```python
from build123d import *

# Parameters (mm, degrees)
BOSS_EXTRUDE1_DEPTH = 45.72
CUT_EXTRUDE1_REACH  = 94.812
SKETCH2_R           = 12.7
SKETCH4_R           = 19.05
CUT_EXTRUDE2_DEPTH  = 2.54
SKETCH5_R           = 1.651
CUT_EXTRUDE3_DEPTH  = 94.150493289
FILLET1_R           = 0.508


with BuildPart() as part:
    # Sketch1 → Boss-Extrude1 (new body)
    with BuildSketch(Plane.XY):
        Polygon((13.1, 7.855), (5.48, 7.855), (5.48, 3.81), (80.52, 3.81), (80.52, 7.855), (72.9, 7.855), (72.9, 10.16), (13.1, 10.16), align=None)
    extrude(amount=-BOSS_EXTRUDE1_DEPTH)

    # Sketch2 → Cut-Extrude1 (cut, up to next)
    with BuildSketch(Plane.XZ.offset(-3.81), mode=Mode.PRIVATE) as cut_extrude1_sk1:
        with Locations(Location((43, -22.86, 0), (0, 0, 270))):
            Circle(SKETCH2_R)
    cut_extrude1_tool1 = extrude(cut_extrude1_sk1.sketch, amount=-CUT_EXTRUDE1_REACH, mode=Mode.PRIVATE) & part.part
    add(cut_extrude1_tool1.solids().sort_by_distance((43, 3.81, -22.86))[0], mode=Mode.SUBTRACT)

    # Sketch4 → Cut-Extrude2 (cut)
    with BuildSketch(Plane.XZ.offset(-3.81)):
        with Locations(Location((43, -22.86, 0), (0, 0, 270))):
            Circle(SKETCH4_R)
    extrude(amount=-CUT_EXTRUDE2_DEPTH, mode=Mode.SUBTRACT)

    # Sketch5 → Cut-Extrude3 (cut, through all)
    with BuildSketch(Plane.XY):
        with Locations((43, 8.255)):
            Circle(SKETCH5_R)
    extrude(amount=-CUT_EXTRUDE3_DEPTH, mode=Mode.SUBTRACT)

    # Fillet1
    # the kernel refuses this fillet: 0.508 mm, written as the material it adds along each edge
    with BuildSketch(Plane(origin=(43, 6.35, -22.86), x_dir=(0, 0, -1), z_dir=(-1, 0, 0))) as fillet1_piece_1:
        with BuildLine():
            CenterArc((19.05 - FILLET1_R, FILLET1_R), FILLET1_R, 270, 90)
            Line((19.05 - FILLET1_R, 0), (19.05, 0))
            Line((19.05, 0), (19.05, FILLET1_R))
        make_face()
    revolve(axis=Axis((43, 6.35, -22.86), (0, -1, 0)))
    with BuildSketch(Plane(origin=(72.9, 7.855, 0), x_dir=(0, 1, 0), z_dir=(0, 0, -1)), Plane(origin=(13.1, 7.855, 0), x_dir=(-1, 0, 0), z_dir=(0, 0, -1))) as fillet1_piece_2:
        with BuildLine():
            CenterArc((FILLET1_R, FILLET1_R), FILLET1_R, 180, 90)
            Line((0, FILLET1_R), (0, 0))
            Line((0, 0), (FILLET1_R, 0))
        make_face()
    extrude(amount=45.72)
    # the kernel refuses this fillet: 0.508 mm, written as the material it takes off along each edge
    with BuildSketch(Plane(origin=(72.9, 8.363, -45.72), x_dir=(-1, 0, 0), z_dir=(0, 1, 0)), Plane(origin=(13.1, 11.43, -45.72), x_dir=(1, 0, 0), z_dir=(0, -1, 0))) as fillet1_2_piece_1:
        with BuildLine():
            CenterArc((FILLET1_R, FILLET1_R), FILLET1_R, 180, 90)
            Line((0, FILLET1_R), (0, 0))
            Line((0, 0), (FILLET1_R, 0))
        make_face()
    extrude(amount=3.067, mode=Mode.SUBTRACT)
    with BuildSketch(Plane(origin=(72.9, 8.363, 0), x_dir=(-1, 0, 0), z_dir=(0, 1, 0)), Plane(origin=(13.1, 11.43, 0), x_dir=(1, 0, 0), z_dir=(0, -1, 0))) as fillet1_2_piece_2:
        with BuildLine():
            CenterArc((FILLET1_R, -FILLET1_R), FILLET1_R, 90, 90)
            Line((0, -FILLET1_R), (0, 0))
            Line((0, 0), (FILLET1_R, 0))
        make_face()
    extrude(amount=3.067, mode=Mode.SUBTRACT)
    with BuildSketch(Plane(origin=(43, 6.35, -22.86), x_dir=(0, 0, -1), z_dir=(-1, 0, 0))) as fillet1_2_piece_3:
        with BuildLine():
            CenterArc((12.7 + FILLET1_R, -FILLET1_R), FILLET1_R, 90, 90)
            Line((12.7 + FILLET1_R, 0), (12.7, 0))
            Line((12.7, 0), (12.7, -FILLET1_R))
        make_face()
    revolve(axis=Axis((43, 6.35, -22.86), (0, -1, 0)), mode=Mode.SUBTRACT)
    with BuildSketch(Plane(origin=(4.21, 3.81, -45.72), x_dir=(0, 1, 0), z_dir=(1, 0, 0))) as fillet1_2_piece_4:
        with BuildLine():
            CenterArc((FILLET1_R, FILLET1_R), FILLET1_R, 180, 90)
            Line((0, FILLET1_R), (0, 0))
            Line((0, 0), (FILLET1_R, 0))
        make_face()
    extrude(amount=77.58, mode=Mode.SUBTRACT)
    with BuildSketch(Plane(origin=(4.21, 3.81, 0), x_dir=(0, 1, 0), z_dir=(1, 0, 0))) as fillet1_2_piece_5:
        with BuildLine():
            CenterArc((FILLET1_R, -FILLET1_R), FILLET1_R, 90, 90)
            Line((0, -FILLET1_R), (0, 0))
            Line((0, 0), (FILLET1_R, 0))
        make_face()
    extrude(amount=77.58, mode=Mode.SUBTRACT)
    with BuildSketch(Plane(origin=(81.79, 7.855, -45.72), x_dir=(0, -1, 0), z_dir=(-1, 0, 0)), Plane(origin=(12.592, 7.855, 0), x_dir=(0, 0, -1), z_dir=(-1, 0, 0))) as fillet1_2_piece_6:
        with BuildLine():
            CenterArc((FILLET1_R, FILLET1_R), FILLET1_R, 180, 90)
            Line((0, FILLET1_R), (0, 0))
            Line((0, 0), (FILLET1_R, 0))
        make_face()
    extrude(amount=8.382, mode=Mode.SUBTRACT)
    with BuildSketch(Plane(origin=(81.79, 7.855, 0), x_dir=(0, -1, 0), z_dir=(-1, 0, 0)), Plane(origin=(12.592, 7.855, -45.72), x_dir=(0, 0, 1), z_dir=(-1, 0, 0))) as fillet1_2_piece_7:
        with BuildLine():
            CenterArc((FILLET1_R, -FILLET1_R), FILLET1_R, 90, 90)
            Line((0, -FILLET1_R), (0, 0))
            Line((0, 0), (FILLET1_R, 0))
        make_face()
    extrude(amount=8.382, mode=Mode.SUBTRACT)
    with BuildSketch(Plane(origin=(72.9, 10.16, 1.27), x_dir=(-1, 0, 0), z_dir=(0, 0, -1)), Plane(origin=(13.1, 10.16, 1.27), x_dir=(0, -1, 0), z_dir=(0, 0, -1))) as fillet1_2_piece_8:
        with BuildLine():
            CenterArc((FILLET1_R, -FILLET1_R), FILLET1_R, 90, 90)
            Line((0, -FILLET1_R), (0, 0))
            Line((0, 0), (FILLET1_R, 0))
        make_face()
    extrude(amount=48.26, mode=Mode.SUBTRACT)
    with BuildSketch(Plane(origin=(43, 10.16, -22.86), x_dir=(0, 0, -1), z_dir=(-1, 0, 0))) as fillet1_2_piece_9:
        with BuildLine():
            CenterArc((12.7 + FILLET1_R, FILLET1_R), FILLET1_R, 180, 90)
            Line((12.7, FILLET1_R), (12.7, 0))
            Line((12.7, 0), (12.7 + FILLET1_R, 0))
        make_face()
    revolve(axis=Axis((43, 10.16, -22.86), (0, -1, 0)), mode=Mode.SUBTRACT)
    with BuildSketch(Plane(origin=(12.592, 8.363, 0), x_dir=(0, -1, 0), z_dir=(-1, 0, 0))) as fillet1_2_piece_10:
        with BuildLine():
            CenterArc((0.508 + FILLET1_R, -FILLET1_R), FILLET1_R, 90, 90)
            Line((0.508, -FILLET1_R), (0.508, 0))
            Line((0.508, 0), (0.508 + FILLET1_R, 0))
        make_face()
    revolve(axis=Axis((12.592, 8.363, 0), (0, 0, 1)), revolution_arc=90, mode=Mode.SUBTRACT)
    with BuildSketch(Plane(origin=(12.592, 8.363, -45.72), x_dir=(0, -1, 0), z_dir=(-1, 0, 0))) as fillet1_2_piece_11:
        with BuildLine():
            CenterArc((0.508 + FILLET1_R, FILLET1_R), FILLET1_R, 180, 90)
            Line((0.508, FILLET1_R), (0.508, 0))
            Line((0.508, 0), (0.508 + FILLET1_R, 0))
        make_face()
    revolve(axis=Axis((12.592, 8.363, -45.72), (0, 0, 1)), revolution_arc=90, mode=Mode.SUBTRACT)
    with BuildSketch(Plane(origin=(73.408, 8.363, 0), x_dir=(-1, 0, 0), z_dir=(0, 1, 0))) as fillet1_2_piece_12:
        with BuildLine():
            CenterArc((0.508 + FILLET1_R, -FILLET1_R), FILLET1_R, 90, 90)
            Line((0.508, -FILLET1_R), (0.508, 0))
            Line((0.508, 0), (0.508 + FILLET1_R, 0))
        make_face()
    revolve(axis=Axis((73.408, 8.363, 0), (0, 0, 1)), revolution_arc=90, mode=Mode.SUBTRACT)
    with BuildSketch(Plane(origin=(73.408, 8.363, -45.72), x_dir=(-1, 0, 0), z_dir=(0, 1, 0))) as fillet1_2_piece_13:
        with BuildLine():
            CenterArc((0.508 + FILLET1_R, FILLET1_R), FILLET1_R, 180, 90)
            Line((0.508, FILLET1_R), (0.508, 0))
            Line((0.508, 0), (0.508 + FILLET1_R, 0))
        make_face()
    revolve(axis=Axis((73.408, 8.363, -45.72), (0, 0, 1)), revolution_arc=90, mode=Mode.SUBTRACT)


solid = part.part
```
Part model, mm, in its own coordinate system. A direction names the side the tool comes from. Round coordinates to 2 decimals unless told otherwise and drop trailing zeros. Write each loop counter-clockwise with the first axis right and the second up, starting at its lowest first coordinate (ties: lowest second). Pieces come first, ordered by that corner, then holes. Notation, with made-up numbers: M -12.75,40.25 L 33.25,40.25 A27 cw 33.25,72.25 Z; hole C 66,85.25 d5. An arc over 180 degrees is marked long. Answer as CSV lines item,"result". Start each with the question number.
1) Drop flat-ended pins along their axis: pin 1 (8 mm diameter, centred on x = 76, z = -21, fed in from +Y); pin 2 (8 mm diameter, centred on x = 9.5, z = -29, fed in from +Y); pin 3 (0.6 mm diameter, centred on y = 9, z = -14.5, fed in from +X). Give the stop position or say it passes through.
2) Mould opens along X. For faces 1 (the face through (55.697, 8.235, -23.127)), 2 (the face through (80.52, 6, -23)), 3 (the face through (26, 3.81, -13)) say: +X half, -X half, draft (parallel to the pull), parting line (faces both ways), or undercut.
3) Band-saw the part on A-A (z = -22.86). List the corners of the cut face in (x, y) (3 decimals).
4) Drill centre lines: L1, parallel to Y at x = 43, z = -39; L2, parallel to X at y = 5.35, z = -22.86; L3, parallel to Y at x = 57, z = -10.5. Where is each one in solid material? Low to high.
5) Which spindle directions (+Z, -Z, +X, -X, +Y, -Y) get a long thin tool onto all of the face, cutting with end or side? Do faces 4 (the face through (9, 7.855, -23)), 5 (the face through (30.303, 8.235, -22.593)), 6 (the face through (77, 7.855, -23)), 7 (the face through (44, 6, -45.72)), 8 (the face through (47, 6.35, -10)). Say none if no direction does.
6) Band-saw the part on B-B (x = 43). List the corners of the cut face in (y, z), then the cut area to 3 significant figures.
Worked out:
1,pin 1,"y = 10.16"
1,pin 2,"y = 10.15"
1,pin 3,"x = 72.9"
2,face 1,"undercut"
2,face 2,"+X half"
2,face 3,"draft"
3,outline,"M 5.48,3.81 L 23.95,3.81 L 23.95,5.842 A0.508 cw 24.458,6.35 L 29.792,6.35 A0.508 ccw 30.3,6.858 L 30.3,9.652 A0.508 ccw 29.792,10.16 L 13.608,10.16 A0.508 ccw 13.1,9.652 L 13.1,8.363 A0.508 cw 12.592,7.855 L 5.48,7.855 Z; M 55.7,6.858 A0.508 ccw 56.208,6.35 L 61.542,6.35 A0.508 cw 62.05,5.842 L 62.05,3.81 L 80.52,3.81 L 80.52,7.855 L 73.408,7.855 A0.508 cw 72.9,8.363 L 72.9,9.652 A0.508 ccw 72.392,10.16 L 56.208,10.16 A0.508 ccw 55.7,9.652 Z"
4,L1,"6.35 to 6.6, 9.91 to 10.16"
4,L2,"5.48 to 23.95, 62.05 to 80.52"
4,L3,"6.33 to 10.16"
5,face 4,"+Z, -Z, -X, +Y"
5,face 5,"+Y, -Y"
5,face 6,"+Z, -Z, +X, +Y"
5,face 7,"-Z, +X, -X, +Y, -Y"
5,face 8,"-Y"
6,outline,"M 3.81,-45.21 A0.51 ccw 4.32,-45.72 L 6.6,-45.72 L 6.6,-35.63 A0.51 ccw 6.35,-36.07 L 6.35,-41.4 A0.51 cw 5.84,-41.91 L 3.81,-41.91 Z; M 3.81,-3.81 L 5.84,-3.81 A0.51 cw 6.35,-4.32 L 6.35,-9.65 A0.51 ccw 6.6,-10.09 L 6.6,0 L 4.32,0 A0.51 ccw 3.81,-0.51 Z; M 9.91,-45.72 L 10.16,-45.72 L 10.16,-36.07 A0.51 ccw 9.91,-35.63 Z; M 9.91,-10.09 A0.51 ccw 10.16,-9.65 L 10.16,0 L 9.91,0 Z"
6,area,"29.5 mm²"
